The model under review builds one solid part; all positions refer to its coordinate system, in mm. Give positions to 0.01 mm unless a question says otherwise; leave off trailing zeros. Order: outer loops, then holes, each group sorted by start corner. A loop starts at its lowest first (then second) coordinate and runs counter-clockwise, first axis right, second up. Notation, with made-up numbers: (78.5, 80.25) - (126.5, 80.25) arc R22 cw to (126.5, 113.25) - close; hole circle Ø4 at (-28.75, 14.5). An arc over 180 degrees is marked (long way). Use a Markdown table: item, result. Add a question column.
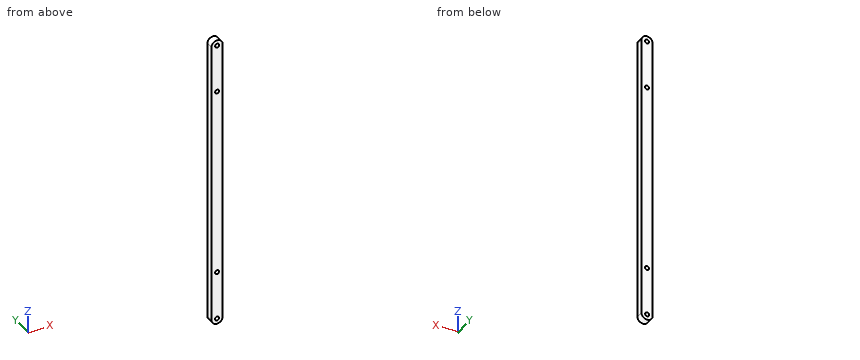
Autodesk Inventor part; units mm, degrees
ref_plane "YZ Plane" through (0, 0, 0) normal (1, 0, 0) x (0, 1, 0)
ref_plane "XZ Plane" through (0, 0, 0) normal (0, 1, 0) x (-1, 0, 0)
ref_plane "XY Plane" through (0, 0, 0) normal (0, 0, 1) x (1, 0, 0)
sketch "Sketch1" plane through (0, 0, 0) normal (0, 1, 0) x (-1, 0, 0)
  line L0 (0, 0) -> (0, -153.89) construction
  line L1 (3, 0) -> (3, -153.89)
  line L2 (-3, -153.89) -> (-3, 0)
  arc A0 (3, 0) -> (-3, 0) centre (0, 0) ccw
  arc A1 (-3, -153.89) -> (3, -153.89) centre (0, -153.89) ccw
  circle A2 centre (0, 0) radius 1.1
  circle A3 centre (0, -153.89) radius 1.1
  circle A4 centre (0, -25.907) radius 1.1
  circle A5 centre (0, -127.773) radius 1.1
  point P0 (0, -76.945)
  dimension "d0" = 2.2
  dimension "d1" = 2.2
  dimension "d2" = 6
  dimension "d3" = 153.89
  dimension "d10" = 2.2
  dimension "d11" = 25.907
  dimension "d12" = 2.2
  dimension "d13" = 127.773
extrude "Extrusion1" add sketch "Sketch1" along normal blind 4
Q1. We need section A-A (x = 0). Write out the cut boundary in (y, z), plus the area to 3 significant figures.
Q2. Clearance check with a flat-ended pin moving along its axis: P1, Ø1.3, axis at x = 0, z = 0, coming from the +Y side. State where the tip first meets the part, or that it passes through.
Q3. Wall thickness on probe 1 along Z at (x, y) = (0, 2.25); probe 2 along Z at (x, y) = (-2.7, 3.6); probe 3 along Z at (x, y) = (1.15, 1.25): over which ranges is each line inside the solid? List them lowest first.
Q4. We need section B-B (y = 1). Write out the cut boundary in (x, z).
Here are the results:
| question | item | result |
|---|---|---|
| 1 | outline | (0, -156.89) - (4, -156.89) - (4, -154.99) - (0, -154.99) - close; (0, -152.79) - (4, -152.79) - (4, -128.87) - (0, -128.87) - close; (0, -126.67) - (4, -126.67) - (4, -27.01) - (0, -27.01) - close; (0, -24.81) - (4, -24.81) - (4, -1.1) - (0, -1.1) - close; (0, 1.1) - (4, 1.1) - (4, 3) - (0, 3) - close |
| 1 | area | 604 mm2 |
| 2 | P1 | through |
| 3 | probe 1 | -156.89 to -154.99, -152.79 to -128.87, -126.67 to -27.01, -24.81 to -1.1, 1.1 to 3 |
| 3 | probe 2 | -155.2 to 1.31 |
| 3 | probe 3 | -156.66 to 2.77 |
| 4 | outline | (-3, -153.89) arc R3 ccw to (3, -153.89) - (3, 0) arc R3 ccw to (-3, 0) - close; hole circle Ø2.2 at (0, -153.89); hole circle Ø2.2 at (0, -127.77); hole circle Ø2.2 at (0, -25.91); hole circle Ø2.2 at (0, 0) |
